The listing builds one solid part. Answer for the finished solid, in the listing's coordinates (mm). Give positions to 0.01 mm unless a question says otherwise; leave off trailing zeros. Order: outer loops, then holes, each group sorted by start corner. A loop starts at its lowest first (then second) coordinate and runs counter-clockwise, first axis right, second up. Notation, with made-up numbers: (28, -38) - (71, -38) arc R24 ccw to (71, -5) - close; hole circle Ø4 at (27.5, 89). An arc over 180 degrees is marked (long way). Use a Markdown table: item, result. Add a question column.
1) Find section C-C, the plane y = 76.2. Determine the outline of the cut face in (x, z).
2) Find section A-A, the plane x = 0. Determine the outline of the cut face in (y, z) (3 decimals), plus the area to 3 significant figures.
3) Straight lines are drawn through the part: line 1 (Y direction, x = 52.5, z = 0.1); line 2 (Y direction, x = 120, z = 0.05); line 3 (Y direction, x = -107.95, z = 0.05). For each, find the intervals that lie inside material, in ascending order.
4) Find section B-B, the plane y = 0. State how many separate pieces and enclosed holes the cut face has, plus the area to 3 significant figures.
5) Find section D-D, the plane y = -38.1. Determine the outline of the cut face in (x, z), plus the area to 3 significant figures.
from build123d import *

# Parameters (mm, degrees)
F0_R     = 152.4
F1_DEPTH = 0.14732
F2_W     = 12.7
F2_H     = 127
F2_W_2   = 127
F2_H_2   = 12.7
F3_DEPTH = 25.4
F5_D     = 6.858
F6_W     = 7.5
F6_H     = 7.5
F7_DEPTH = 25.4


with BuildPart() as f1:
    # F0 (on Top) → F1 (new body)
    with BuildSketch(Plane.XY):
        Circle(F0_R)
    extrude(amount=F1_DEPTH)

    # F2 (on face) → F3 (cut)
    with BuildSketch(Plane.XY.offset(0.14732)):
        with Locations((-155.575, 0)):
            Rectangle(F2_W, F2_H)
        with Locations((0, -155.575)):
            Rectangle(F2_W_2, F2_H_2)
        with Locations((0, 155.575)):
            Rectangle(F2_W_2, F2_H_2)
        with Locations((155.575, 0)):
            Rectangle(F2_W, F2_H)
    extrude(amount=-F3_DEPTH, mode=Mode.SUBTRACT)

    # F5 (through all)
    with Locations(Plane.XY.offset(0.14732)):
        with Locations((-53.868412, -93.672059), (54.294765, -93.672059), (65.991136, -38.1), (0, -38.1), (-65.991136, -38.1), (-107.95, 0), (-32.995568, 19.05), (32.995568, 19.05), (108.376353, 0), (0, 76.2), (54.294765, 93.672059), (-53.868412, 93.672059)):
            Hole(F5_D / 2)

    # F6 (on face) → F7 (cut)
    with BuildSketch(Plane.XY.offset(0.14732)):
        Rectangle(F6_W, F6_H)
        with Locations((-63.4965, 0)):
            Rectangle(F6_W, F6_H)
        with Locations((0, 110.109)):
            Rectangle(F6_W, F6_H)
        Polygon((-36.870845, -56.362177), (-30.375655, -60.112177), (-26.625655, -53.616987), (-33.120845, -49.866987), align=None)
        Polygon((30.375655, -60.112177), (36.870845, -56.362177), (33.120845, -49.866987), (26.625655, -53.616987), align=None)
        with Locations((63.4965, 0)):
            Rectangle(F6_W, F6_H)
        Polygon((36.870845, 56.362177), (30.375655, 60.112177), (26.625655, 53.616987), (33.120845, 49.866987), align=None)
        Polygon((-30.375655, 60.112177), (-36.870845, 56.362177), (-33.120845, 49.866987), (-26.625655, 53.616987), align=None)
        Polygon((-100.479786, 53.681905), (-93.984596, 49.931905), (-90.234596, 56.427095), (-96.729786, 60.177095), align=None)
        Polygon((-96.729786, -60.177095), (-90.234596, -56.427095), (-93.984596, -49.931905), (-100.479786, -53.681905), align=None)
        with Locations((0, -110.109)):
            Rectangle(F6_W, F6_H)
        Polygon((100.479786, -53.681905), (93.984596, -49.931905), (90.234596, -56.427095), (96.729786, -60.177095), align=None)
        Polygon((96.729786, 60.177095), (90.234596, 56.427095), (93.984596, 49.931905), (100.479786, 53.681905), align=None)
    extrude(amount=-F7_DEPTH, mode=Mode.SUBTRACT)


solid = f1.part
The answers:
| question | item | result |
|---|---|---|
| 1 | outline | (-131.98, 0) - (-3.43, 0) - (-3.43, 0.15) - (-131.98, 0.15) - close; (3.43, 0) - (131.98, 0) - (131.98, 0.15) - (3.43, 0.15) - close |
| 2 | outline | (-149.225, 0) - (-113.859, 0) - (-113.859, 0.147) - (-149.225, 0.147) - close; (-106.359, 0) - (-41.529, 0) - (-41.529, 0.147) - (-106.359, 0.147) - close; (-34.671, 0) - (-3.75, 0) - (-3.75, 0.147) - (-34.671, 0.147) - close; (3.75, 0) - (72.771, 0) - (72.771, 0.147) - (3.75, 0.147) - close; (79.629, 0) - (106.359, 0) - (106.359, 0.147) - (79.629, 0.147) - close; (113.859, 0) - (149.225, 0) - (149.225, 0.147) - (113.859, 0.147) - close |
| 2 | area | 38.6 mm2 |
| 3 | line 1 | -143.07 to -96.59, -90.75 to 90.75, 96.59 to 143.07 |
| 3 | line 2 | -93.95 to 93.95 |
| 3 | line 3 | -107.58 to -3.43, 3.43 to 107.58 |
| 4 | separate pieces | 6 |
| 4 | enclosed holes | 0 |
| 4 | area | 38.6 mm2 |
| 5 | outline | (-147.56, 0) - (-69.42, 0) - (-69.42, 0.15) - (-147.56, 0.15) - close; (-62.56, 0) - (-3.43, 0) - (-3.43, 0.15) - (-62.56, 0.15) - close; (3.43, 0) - (62.56, 0) - (62.56, 0.15) - (3.43, 0.15) - close; (69.42, 0) - (147.56, 0) - (147.56, 0.15) - (69.42, 0.15) - close |
| 5 | area | 40.4 mm2 |
